The listing builds one solid part. Answer for the finished solid, in the listing's coordinates (mm). A direction names the side the tool comes from. Give positions to 0.01 mm unless a question says otherwise; leave off trailing zeros. Write each loop counter-clockwise with the first axis right and the second up, starting at its lowest first coordinate (ties: lowest second). Pieces come first, ordered by that corner, then holes. Notation, with made-up numbers: (87, -20.5) -> (93, -20.5) arc R20 ccw to (93, 4.5) -> close; hole circle Ø6 at (-21, 35). An arc over 180 degrees is marked (long way). One line per question, with ' | ' between items.
Autodesk Inventor part; units mm, degrees
ref_plane "YZ Plane" through (0, 0, 0) normal (1, 0, 0) x (0, 1, 0)
ref_plane "XZ Plane" through (0, 0, 0) normal (0, 1, 0) x (-1, 0, 0)
ref_plane "XY Plane" through (0, 0, 0) normal (0, 0, 1) x (1, 0, 0)
sketch "Sketch1" plane through (0, 0, 0) normal (0, 0, 1) x (1, 0, 0)
  circle A0 centre (0, 0) radius 3
  line L0 (-1.4524, 2.625) -> (1.4524, 2.625)
  line L1 (-4.1421, -10) -> (-10, -4.1421)
  line L2 (-10, -4.1421) -> (-10, 4.1421)
  line L3 (-10, 4.1421) -> (-4.1421, 10)
  line L4 (-4.1421, 10) -> (4.1421, 10)
  line L5 (4.1421, 10) -> (10, 4.1421)
  line L6 (10, 4.1421) -> (10, -4.1421)
  line L7 (10, -4.1421) -> (4.1421, -10)
  line L8 (4.1421, -10) -> (-4.1421, -10)
  circle A1 centre (29.944, -1.8315) radius 1.5
  circle A2 centre (29.944, 1.8315) radius 1.5
  circle A3 centre (0, 0) radius 30 construction
  line L9 (0, 0) -> (30, 0) construction
  line L10 (0, 0) -> (29.944, 1.8315) construction
  line L11 (0, 0) -> (29.944, -1.8315) construction
  circle A4 centre (0, 0) radius 40 construction
  circle A5 centre (39.7623, 4.3547) radius 1.5
  circle A6 centre (40, 0) radius 1.5
  circle A7 centre (39.7623, -4.3547) radius 1.5
  line L12 (0, 0) -> (39.7623, 4.3547) construction
  line L13 (40, 0) -> (0, 0) construction
  line L14 (0, 0) -> (39.7623, -4.3547) construction
  circle A8 centre (50, 0) radius 1.5
  circle A9 centre (65, 0) radius 1.5
  circle A10 centre (-5.5, 0) radius 1.5
  line L15 (0, 0) -> (65, 0) construction
  line L16 (0, -10) -> (65, -10)
  line L17 (65, 10) -> (0, 10)
  arc A11 (0, 10) -> (0, -10) centre (0, 0) ccw
  arc A12 (65, -10) -> (65, 10) centre (65, 0) ccw
  line L18 (0, 10) -> (-10, 10)
  line L19 (-10, 10) -> (-10, -10)
  line L20 (-10, -10) -> (0, -10)
  line L21 (0, -10) -> (0, 10)
  line L22 (65, 10) -> (75, 10)
  line L23 (75, 10) -> (75, -10)
  line L24 (75, -10) -> (65, -10)
  line L25 (65, -10) -> (65, 10)
  point P0 (32.5, 0)
  point P1 (4.1421, -10)
  point P2 (0, 10)
  point P3 (0, 0)
  point P4 (65, 0)
  point P5 (75, 0)
  point P6 (-10, 0)
  dimension "d0" = 6
  dimension "d1" = 2.625
  dimension "d2" = 20
  dimension "d3" = 3
  dimension "d4" = 3
  dimension "d5" = 60
  dimension "d6" = 3.5
  dimension "d7" = 3.5
  dimension "d8" = 80
  dimension "d9" = 3
  dimension "d10" = 3
  dimension "d11" = 3
  dimension "d12" = 0
  dimension "d13" = 6.25
  dimension "d14" = 6.25
  dimension "d15" = 3
  dimension "d16" = 3
  dimension "d17" = 0
  dimension "d18" = 50
  dimension "d19" = 0
  dimension "d20" = 65
  dimension "d21" = 3
  dimension "d22" = 0
  dimension "d23" = 5.5
  dimension "d24" = 20
  dimension "d36" = 10
  dimension "d37" = 10
  dimension "d38" = 20
  dimension "d44" = 10
extrude "Extrusion1" add sketch "Sketch1" along normal blind 3 contours A0 L21 L4 L5 L6 L7 L8 | L0 L21 A0 | L21 A11 A0 | L21 L0 A0 | L8 L1 A11 | A11 L3 L4 | L7 L6 L5 L17 L25 A9 L16 | L20 L19 L1 | L1 L2 A11 | L3 L19 L18 | A11 L2 L3 | L25 A9 A12 | A12 L23 L24 | L22 L23 A12 picked at (0.8147, 2.6938) picked at (-0.8147, 2.6938)
sketch "Sketch2" plane through (0, 0, 3) normal (0, 0, 1) x (1, 0, 0)
  line L0 (75, 10) -> (-10, 10)
  line L1 (-10, -10) -> (75, -10)
  line L2 (25, 10) -> (55, 10)
  line L3 (55, 10) -> (55, -10)
  line L4 (55, -10) -> (25, -10)
  line L5 (25, -10) -> (25, 10)
  line L6 (25, 6) -> (-9, 6)
  line L7 (-9, 6) -> (-9, -6)
  line L8 (-9, -6) -> (25, -6)
  line L9 (25, -6) -> (25, 6)
  line L10 (55, 6) -> (75, 6)
  line L11 (75, 6) -> (75, -6)
  line L12 (75, -6) -> (55, -6)
  line L13 (55, -6) -> (55, 6)
  circle A0 centre (65, 0) radius 1.5
  line L14 (75, 10) -> (-10, 10)
  line L15 (-10, 10) -> (-10, -10)
  line L16 (-10, -10) -> (75, -10)
  line L17 (75, -10) -> (75, 10)
  arc A1 (-1.4524, 2.625) -> (1.4524, 2.625) centre (0, 0) ccw
  circle A2 centre (29.944, -1.8315) radius 1.5
  circle A3 centre (29.944, 1.8315) radius 1.5
  circle A4 centre (39.7623, 4.3547) radius 1.5
  circle A5 centre (40, 0) radius 1.5
  circle A6 centre (39.7623, -4.3547) radius 1.5
  circle A7 centre (50, 0) radius 1.5
  circle A8 centre (65, 0) radius 1.5
  line L18 (-1.4524, 2.625) -> (1.4524, 2.625)
  point P0 (-9, 0)
  point P1 (55, -6)
  point P2 (-10, -6)
  point P3 (-10, -10)
  point P4 (25, -6)
  point P5 (-10, 6)
  dimension "d28" = 6
  dimension "d29" = 6
  dimension "d30" = 9
  dimension "d31" = 6
  dimension "d32" = 10
  dimension "d33" = 6
  dimension "d34" = 10
  dimension "d39" = 25
extrude "Extrusion2" cut sketch "Sketch2" against normal up to surface (3 mm away) contours L17 L10 L3 L0 | L5 L6 L7 L8 L1 L15 L0 | L17 L1 L3 L12
fillet "Fillet1" radius 2 8 edges at (25, -6, 1.5) (25, -10, 1.5) (55, -10, 1.5) (55, -6, 1.5) (25, 10, 1.5) (25, 6, 1.5) (55, 10, 1.5) (55, 6, 1.5)
fillet "Fillet1" radius 6 4 edges at (75, 6, 1.5) (75, -6, 1.5) (-9, 6, 1.5) (-9, -6, 1.5)
equation "\"d7\" = d6"
equation "\"d14\" = d13"
equation "\"d31\" = d28"
equation "\"d33\" = d28"
properties part number "Arm1" material "Aluminum 6061, Welded"
Item 1: A tool of negligible diameter and unlimited length cuts with its end or side. For faces 1 (the face through (0, 2.625, 1)), 2 (the face through (10, 6, 2)), 3 (the face through (10, -6, 2)), from which of +Z, -Z, +X, -X, +Y, -Y can it reach the whole face along a straight path? Write none if from no direction.
Answers below:
face 1: +Z, -Z | face 2: +Z, -Z, -X, +Y | face 3: +Z, -Z, -X, -Y
Item 2: Find section D-D (x = 40). Write down the section's boundary in (y, z), then the cut area to 3 significant figures.
Answers below:
outline: (-10, 0) -> (-5.84, 0) -> (-5.84, 3) -> (-10, 3) -> close; (-2.87, 0) -> (-1.5, 0) -> (-1.5, 3) -> (-2.87, 3) -> close; (1.5, 0) -> (2.87, 0) -> (2.87, 3) -> (1.5, 3) -> close; (5.84, 0) -> (10, 0) -> (10, 3) -> (5.84, 3) -> close | area: 33.2 mm²
Item 3: Find section B-B (x = 65). Write down the section's boundary in (y, z).
Answers below:
outline: (-6, 0) -> (-1.5, 0) -> (-1.5, 3) -> (-6, 3) -> close; (1.5, 0) -> (6, 0) -> (6, 3) -> (1.5, 3) -> close
Item 4: Find section C-C (z = 1.2). Count the separate pieces of the cut face and the enclosed holes in it, then the cut area to 3 significant figures.
Answers below:
separate pieces: 1 | enclosed holes: 9 | area: 1,130 mm²
Item 5: Find section A-A (x = 50). Write down the section's boundary in (y, z), then the cut area to 3 significant figures.
Answers below:
outline: (-10, 0) -> (-1.5, 0) -> (-1.5, 3) -> (-10, 3) -> close; (1.5, 0) -> (10, 0) -> (10, 3) -> (1.5, 3) -> close | area: 51.0 mm²
Item 6: Consider line 1 (Y direction, x = 40, z = 1.75); line 2 (X direction, y = -2.5, z = 2.55); line 3 (Y direction, x = 17.5, z = 2.7). Determine where each line is inside the solid, lowest interval first. Write a range as [from, to].
Answers below:
line 1: [-10, -5.84], [-2.87, -1.5], [1.5, 2.87], [5.84, 10] | line 2: [-8.45, -1.66], [1.66, 28.6], [31.29, 74.45] | line 3: [-6, 6]
Item 7: Flat-ended cylindrical pins translate along their axes: pin 1 (5 mm diameter, centred on x = 50, y = 0, fed in from -Z); pin 2 (1.5 mm diameter, centred on x = -0.5, z = 2, fed in from -Y); pin 3 (1.5 mm diameter, centred on x = 13, z = 2, fed in from +Y). Find the tip coordinate at first contact, or state that the pin passes through.
Answers below:
pin 1: z = 0 | pin 2: y = -6 | pin 3: y = 6
